Geometry check sheet. Reference: the model listing, model coordinates, mm. A direction names the side the tool comes from. Coordinates: 2 decimals unless noted, no trailing zeros. Write each loop counter-clockwise with the first axis right and the second up, starting at its lowest first coordinate (ties: lowest second). Pieces come first, ordered by that corner, then holes. Notation, with made-up numbers: (-3, -8.75) -> (43, -8.75) arc R21 ccw to (43, -2.75) -> close; hole circle Ø10 at (-6, 49). An arc over 180 degrees is marked (long way). Answer in a Markdown table with one row per item. Add a question column.
1. Cross-section at C-C on y = -22. Record the cut outline in (x, z).
2. Mould release check, pull along Z, two halves, no side actions. Record for faces 4 (the flat face through (41, -11, -19)), 5 (the flat face through (14, 2, 80)), 6 (the cylindrical face through (54.4, 0.06, 31.67)), 7 (the flat face through (-24, -2, 29)): pulls with the +Z half, pulls with the -Z half, needs draft (parallel to the pull), parting line crosses it, or undercut.
3. Depth check by flat-ended pin: P1, Ø2, axis at x = 49, y = -1.5, coming from the +Z side; P2, Ø15.5, axis at x = -7.5, z = 32, coming from the -Y side; P3, Ø1, axis at x = 3.5, z = -8.5, coming from the +Y side. Enter the tip coordinate at first touch or a pass-through.
4. Scan lines: L1, parallel to Z at x = -7, y = -1.5; L2, parallel to X at y = -1, z = 15.5; L3, parallel to X at y = 2.2, z = -22.5. Record each from-to range of solid material in increasing order. Write a range as from..to.
5. Cross-section at A-A on z = -47.5. Record the cut outline in (x, y).
6. Set-up check for faces 1 (the flat face through (-21.989, -2.028, 35.915)), 2 (the flat face through (56.693, -2, 31)), 3 (the flat face through (34.282, 0, 31)): record each of +Z, -Z, +X, -X, +Y, -Y from which the full face is reachable in a straight line by a thin tool's end or side.
7. Cross-section at D-D on x = 13. Record the cut outline in (y, z), and give its area (3 significant figures).
8. Cross-section at B-B on z = 64. Record the cut outline in (x, y), and give its area (3 significant figures).
Autodesk Inventor part; units mm, degrees
ref_plane "YZ Plane" through (0, 0, 0) normal (1, 0, 0) x (0, 1, 0)
ref_plane "XZ Plane" through (0, 0, 0) normal (0, 1, 0) x (-1, 0, 0)
ref_plane "XY Plane" through (0, 0, 0) normal (0, 0, 1) x (1, 0, 0)
sketch "Szkic1" plane through (0, 0, 0) normal (0, 1, 0) x (-1, 0, 0)
  line L0 (44.7185, 35) -> (76.7185, 35)
  line L1 (76.7185, 35) -> (44.7185, 35)
  line L2 (44.7185, -65) -> (76.7185, -65)
  line L3 (76.7185, -65) -> (76.7185, 35)
  line L4 (44.7185, 80) -> (-75.2815, 80)
  line L5 (44.7185, 48) -> (44.7185, 80)
  line L6 (44.7185, -65) -> (44.7185, -55)
  line L7 (-75.2815, -65) -> (-75.2815, 48)
  line L8 (44.7185, -65) -> (-75.2815, -65)
  line L9 (-75.2815, 48) -> (-65.2815, 48)
  line L10 (-75.2815, 48) -> (-75.2815, 80)
  line L11 (44.7185, 35) -> (44.7185, -55)
  line L12 (-65.2815, -55) -> (44.7185, -55)
  line L13 (-65.2815, -55) -> (-65.2815, 48)
  line L14 (44.7185, 48) -> (-65.2815, 48)
  line L15 (44.7185, 35) -> (44.7185, 48)
  point P0 (0, 0)
  point P1 (14.7185, 64)
  point P2 (-45.2815, 64)
  point P3 (60.7185, 2.5)
  point P4 (60.7185, -47.5)
  point P5 (60.7185, -22.5)
  dimension "d2" = 32
  dimension "d3" = 45
  dimension "d4" = 32
  dimension "d5" = 32
  dimension "d23" = 100
  dimension "d24" = 10
  dimension "d25" = 10
  dimension "d26" = 120
  dimension "d27" = 16
  dimension "d28" = 16
  dimension "d29" = 50
  dimension "d30" = 16
  dimension "d31" = 16
  dimension "d32" = 60
  dimension "d33" = 17.5
  dimension "d34" = 30
  dimension "d126" = 42.5
extrude "Wyciągnięcie proste1" add sketch "Szkic1" along normal blind 4
extrude "Wyciągnięcie proste2" add sketch "Szkic1" against normal blind 15 contours L11 L12 L13 L14 L15
extrude "Wyciągnięcie proste3" add sketch "Szkic1" against normal blind 30 contours L6 L8 L7 L9 L13 L12
sketch "Szkic3" plane through (0, 4, 0) normal (0, 1, 0) x (1, 0, 0)
  line L0 (-76.7185, -35) -> (-44.7185, -35)
  line L1 (-44.7185, -35) -> (-44.7185, -80)
  line L2 (-44.7185, -80) -> (75.2815, -80)
  line L3 (75.2815, -80) -> (75.2815, 65)
  line L4 (75.2815, 65) -> (-76.7185, 65)
  line L5 (-76.7185, 65) -> (-76.7185, -35)
  line L6 (-44.7185, -48) -> (75.2815, -48)
  line L7 (-44.7185, 65) -> (-44.7185, -35)
  line L8 (-44.7185, 55) -> (65.2815, 55)
  line L9 (65.2815, 55) -> (65.2815, -48)
  line L10 (-29.7185, -17.5) -> (11.2815, -17.5)
  line L11 (11.2815, -17.5) -> (11.2815, 54.5)
  line L12 (11.2815, 54.5) -> (-29.7185, 54.5)
  line L13 (-29.7185, 54.5) -> (-29.7185, -17.5)
  line L14 (21.2815, -17.5) -> (62.2815, -17.5)
  line L15 (62.2815, -17.5) -> (62.2815, 54.5)
  line L16 (62.2815, 54.5) -> (21.2815, 54.5)
  line L17 (21.2815, 54.5) -> (21.2815, -17.5)
  line L18 (-16.7185, -35.5) -> (-0.7185, -35.5)
  line L19 (-0.7185, -35.5) -> (-0.7185, -26.5)
  line L20 (-0.7185, -26.5) -> (-16.7185, -26.5)
  line L21 (-16.7185, -26.5) -> (-16.7185, -35.5)
  line L22 (-16.7185, -35.5) -> (-0.7185, -26.5) construction
  line L23 (-0.7185, -35.5) -> (-16.7185, -26.5) construction
  circle A0 centre (-19.2185, -31) radius 1.75
  circle A1 centre (1.7815, -31) radius 1.75
  line L24 (-19.2185, -31) -> (1.7815, -31) construction
  circle A2 centre (52.7815, -31) radius 1.75
  line L25 (50.2815, -35.5) -> (50.2815, -26.5)
  line L26 (50.2815, -26.5) -> (34.2815, -26.5)
  line L27 (34.2815, -26.5) -> (34.2815, -35.5)
  line L28 (34.2815, -35.5) -> (50.2815, -26.5) construction
  line L29 (50.2815, -35.5) -> (34.2815, -26.5) construction
  line L30 (34.2815, -35.5) -> (50.2815, -35.5)
  line L31 (31.7815, -31) -> (52.7815, -31) construction
  circle A3 centre (31.7815, -31) radius 1.75
  point P0 (0, 0)
  point P1 (-8.7185, -31)
  point P2 (42.2815, -31)
  dimension "d35" = 41
  dimension "d36" = 72
  dimension "d37" = 41
  dimension "d38" = 72
  dimension "d39" = 10
  dimension "d40" = 15
  dimension "d41" = 30.5
  dimension "d50" = 30.5
  dimension "d78" = 16
  dimension "d79" = 9
  dimension "d80" = 3.5
  dimension "d81" = 3.5
  dimension "d82" = 10.5
  dimension "d83" = 10.5
  dimension "d86" = 4.5
  dimension "d87" = 4.5
  dimension "d88" = 20
  dimension "d89" = 9
  dimension "d90" = 16
  dimension "d91" = 9
  dimension "d92" = 3.5
  dimension "d93" = 3.5
  dimension "d94" = 10.5
  dimension "d95" = 10.5
  dimension "d96" = 4.5
  dimension "d97" = 4.5
  dimension "d102" = 9
  dimension "d127" = 20
extrude "Wyciągnięcie proste4" cut sketch "Szkic3" against normal blind 15 contours L13 L12 L11 L10 | L17 L16 L15 L14
extrude "Wyciągnięcie proste5" cut sketch "Szkic3" against normal blind 20 contours L21 L20 L19 L18 | A0 | A1 | A2 | L30 L27 L26 L25 | A3
sketch "Szkic4" plane through (0, -30, 0) normal (0, -1, 0) x (1, 0, 0)
  line L0 (-44.7185, 48) -> (-44.7185, -55)
  line L1 (-44.7185, -55) -> (65.2815, -55)
  line L2 (65.2815, -55) -> (65.2815, 48)
  line L3 (65.2815, 48) -> (-44.7185, 48)
  line L4 (-44.7185, -55) -> (-44.7185, -65)
  line L5 (-44.7185, -65) -> (75.2815, -65)
  line L6 (75.2815, -65) -> (75.2815, 48)
  line L7 (75.2815, 48) -> (65.2815, 48)
  line L8 (65.2815, 48) -> (65.2815, -55)
  line L9 (65.2815, -55) -> (-44.7185, -55)
  line L10 (65.2815, -55) -> (65.2815, 48)
  line L11 (75.2815, -65) -> (75.2815, 48)
  line L12 (65.2815, -15) -> (75.2815, -15)
  line L13 (75.2815, -15) -> (75.2815, 55)
  line L14 (75.2815, 55) -> (65.2815, 55)
  line L15 (65.2815, 55) -> (65.2815, -15)
  line L16 (-44.7185, -55) -> (65.2815, -55)
  line L17 (25.2815, -55) -> (-44.7185, -55)
  line L18 (-44.7185, -55) -> (-44.7185, -65)
  line L19 (-44.7185, -65) -> (25.2815, -65)
  line L20 (25.2815, -65) -> (25.2815, -55)
  dimension "d111" = 70
  dimension "d112" = 70
  dimension "d113" = 50
  dimension "d114" = 50
extrude "Wyciągnięcie proste6" cut sketch "Szkic4" against normal blind 15 contours L1 L20 L5 L4 | L7 L6 L12 L2 | L15 L14 L13 L7
hole "Otwór1" at (-14.7185, 0, 64) at (45.2815, 0, 64) at (-60.7185, 0, 2.5) at (-60.7185, 0, -47.5) at (-60.7185, 0, -22.5) direction (0, 1, 0) diameter 4.5 end through all
sketch "Szkic5" plane through (0, -15, 0) normal (0, -1, 0) x (1, 0, 0)
  line L0 (-45, 48) -> (-10, 48)
  line L1 (65.2815, 48) -> (-44.7185, 48)
  line L2 (-45, 48) -> (-44.7185, 13.0011)
  line L3 (-44.7185, 13.0011) -> (-10, 48)
  point P0 (0, 0)
  dimension "d74" = 35
extrude "Wyciągnięcie proste7" cut sketch "Szkic5" against normal blind 15
sketch "Szkic6" plane through (75.2815, 0, 80) normal (1, 0, 0) x (0, 0, -1)
  line L0 (145, -30) -> (145, 4)
  line L1 (145, -30) -> (95, -30)
  point P0 (80, 0)
  point P1 (102.5, -22)
  dimension "d117" = 42.5
  dimension "d118" = 8
hole "Otwór2" at (75.2815, -22, -22.5) direction (-1, 0, 0) diameter 4.5 end through all
sketch "Szkic8" plane through (0, -15, 0) normal (0, -1, 0) x (1, 0, 0)
  line L0 (-69, 21) -> (-69, 49)
  line L1 (-69, 49) -> (78, 49)
  line L2 (78, 49) -> (78, 21)
  line L3 (-33, -72) -> (-69, -72)
  line L4 (-69, -72) -> (-69, 21)
  line L5 (-33, 21) -> (-33, -72)
  line L6 (-33, 21) -> (78, 21)
  line L7 (11.2815, 17.5) -> (-29.7185, 17.5)
  line L8 (-29.7185, 17.5) -> (-29.7185, -54.5)
  line L9 (26.8332, 38) -> (56.6926, 38)
  line L10 (56.6926, 38) -> (56.6926, 24)
  line L11 (56.6926, 24) -> (26.8332, 24)
  line L12 (26.8332, 24) -> (26.8332, 38)
  line L13 (6, 38) -> (-24, 38)
  line L14 (-24, 38) -> (-24, 24)
  line L15 (-24, 24) -> (6, 24)
  line L16 (6, 24) -> (6, 38)
  line L17 (-29.7185, -54.5) -> (11.2815, -54.5)
  line L18 (21.2815, -54.5) -> (62.2815, -54.5)
  line L19 (62.2815, -54.5) -> (62.2815, 17.5)
  line L20 (62.2815, 17.5) -> (21.2815, 17.5)
  line L21 (65.2815, -55) -> (65.2815, -15)
  line L22 (78, 21) -> (65.2815, 21)
  line L23 (65.2815, 21) -> (65.2815, -15)
  line L24 (65.2815, -15) -> (78, -15)
  line L25 (78, -15) -> (78, 21)
  point P0 (0, 0)
  point P1 (65.2815, 48)
extrude "Wyciągnięcie proste9" cut sketch "Szkic8" against normal blind 15
sketch "Szkic9" plane through (0, -15, 0) normal (0, -1, 0) x (1, 0, 0)
  line L0 (-28, 43) -> (61, 43)
  line L1 (61, 43) -> (61, 22)
  line L2 (61, 22) -> (-28, 22)
  line L3 (-28, 22) -> (-28, 43)
  point P0 (0, 0)
extrude "Wyciągnięcie proste10" cut sketch "Szkic9" against normal blind 11
equation "\"d4\" = d5"
equation "\"d24\" = d25"
equation "\"d37\" = d35"
equation "\"d38\" = d36"
equation "\"d50\" = d41"
equation "\"d80\" = d84"
equation "\"d81\" = d80"
equation "\"d92\" = d98"
equation "\"d93\" = d92"
equation "\"d102\" = d89"
properties part number "slot na baterie"
Results found:
| question | item | result |
|---|---|---|
| 1 | outline | (25.28, -65) -> (75.28, -65) -> (75.28, -24.75) -> (65.28, -24.75) -> (65.28, -55) -> (25.28, -55) -> close; (65.28, -20.25) -> (75.28, -20.25) -> (75.28, -15) -> (65.28, -15) -> close |
| 2 | face 4 | undercut |
| 2 | face 5 | pulls with the +Z half |
| 2 | face 6 | undercut |
| 2 | face 7 | needs draft |
| 3 | P1 | stops at z = 38 |
| 3 | P2 | stops at y = -4 |
| 3 | P3 | stops at y = -11 |
| 4 | L1 | z = -65..-54.5, 17.5..21, 24..26.5, 35.5..38 |
| 4 | L2 | x = -33..-29.72, 11.28..21.28, 62.28..65.28 |
| 4 | L3 | x = -76.72..-62.97, -58.47..-29.72, 11.28..21.28, 62.28..75.28 |
| 5 | outline | (-76.72, 0) -> (-62.97, 0) -> (-62.97, 4) -> (-76.72, 4) -> close; (-58.47, 0) -> (-33, 0) -> (-33, -15) -> (65.28, -15) -> (65.28, -30) -> (75.28, -30) -> (75.28, 4) -> (62.28, 4) -> (62.28, -11) -> (21.28, -11) -> (21.28, 4) -> (11.28, 4) -> (11.28, -11) -> (-29.72, -11) -> (-29.72, 4) -> (-58.47, 4) -> close |
| 6 | face 1 | +Z, -X, -Y |
| 6 | face 2 | +Z, +X, -Y |
| 6 | face 3 | +Y, -Y |
| 7 | outline | (-15, -65) -> (4, -65) -> (4, 80) -> (0, 80) -> (0, 21) -> (-15, 21) -> close |
| 7 | area | 1,870 mm^2 |
| 8 | outline | (-44.72, 0) -> (-16.97, 0) -> (-16.97, 4) -> (-44.72, 4) -> close; (-12.47, 0) -> (43.03, 0) -> (43.03, 4) -> (-12.47, 4) -> close; (47.53, 0) -> (75.28, 0) -> (75.28, 4) -> (47.53, 4) -> close |
| 8 | area | 444 mm^2 |
